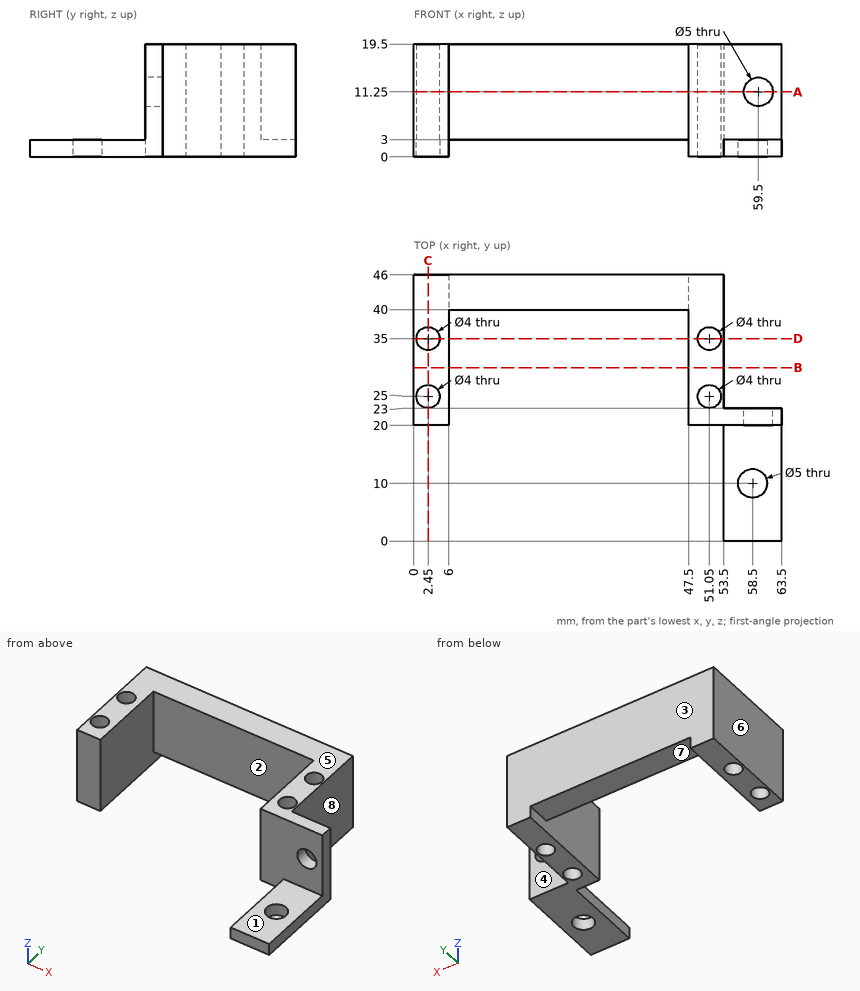
Could you check a few things on this drawing? It's one solid part, dimensions in mm from its lowest x, y, z. A direction names the side the tool comes from. Round coordinates to 2 decimals unless told otherwise and drop trailing zeros. Order: outer loops, then holes, each group sorted by start corner. A loop starts at its lowest first (then second) coordinate and runs counter-clockwise, first axis right, second up. Notation, with made-up numbers: M 5,-24 L 49,-24 A35 cw 49,8 Z; hole C 57.5,18.25 d8. An arc over 180 degrees is marked long. Use a Markdown table: item, result.
1) Imagine slicing it at B-B (y = 30). List the corners of the cut face in (x, z) for me, then the cut area to 3 significant figures.
Geometry says:
| item | result |
|---|---|
| outline | M 0,0 L 6,0 L 6,19.5 L 0,19.5 Z; M 47.5,0 L 53.5,0 L 53.5,19.5 L 47.5,19.5 Z |
| area | 234 mm² |
2) On a 3-axis mill with a long thin cutter (end or side, diameter ignored), from which of +Z, -Z, +X, -X, +Y, -Y can I reach the whole of each face in a straight line? I mean the marked faces 1, 2, 3 and 4. Say none if no direction works.
Geometry says:
| item | result |
|---|---|
| face 1 | +Z, +X, -X, -Y |
| face 2 | +Z, -Z, -Y |
| face 3 | +Z, -Z, +X, -X, +Y |
| face 4 | +Z, -Z, +X, +Y |
3) I'm going to push flat-ended pins straight in: P1, Ø6, axis at x = 17.5, z = 4.5, coming from the -Y side; P2, Ø6.5, axis at x = 30, y = 44, coming from the -Z side; P3, Ø1.8, axis at x = 2.5, z = 9.5, coming from the -Y side. Where does each tip first touch, or does it pass through?
Geometry says:
| item | result |
|---|---|
| P1 | stops at y = 40 |
| P2 | stops at z = 3 |
| P3 | stops at y = 20 |
4) If I drill on line 1 along Y through (x, z) = (2.45, 4.5); line 2 along X through (y, z) = (21.25, 11.25); line 3 along Y through (x, z) = (49, 11), over which ranges is the centre line in solid material (lowest first)?
Geometry says:
| item | result |
|---|---|
| line 1 | y = 20 to 23, 27 to 33, 37 to 46 |
| line 2 | x = 0 to 6, 47.5 to 57, 62 to 63.5 |
| line 3 | y = 20 to 46 |
5) Imagine slicing it at C-C (x = 2.45). List the corners of the cut face in (y, z) for me, then the cut area to 3 significant figures.
Geometry says:
| item | result |
|---|---|
| outline | M 20,0 L 23,0 L 23,19.5 L 20,19.5 Z; M 27,0 L 33,0 L 33,19.5 L 27,19.5 Z; M 37,0 L 46,0 L 46,19.5 L 37,19.5 Z |
| area | 351 mm² |
6) Imagine slicing it at D-D (y = 35). List the corners of the cut face in (x, z) for me, then the cut area to 3 significant figures.
Geometry says:
| item | result |
|---|---|
| outline | M 0,0 L 0.45,0 L 0.45,19.5 L 0,19.5 Z; M 4.45,0 L 6,0 L 6,19.5 L 4.45,19.5 Z; M 47.5,0 L 49.05,0 L 49.05,19.5 L 47.5,19.5 Z; M 53.05,0 L 53.5,0 L 53.5,19.5 L 53.05,19.5 Z |
| area | 78.0 mm² |
7) If we mould it in two halves opening along X, with no side actions, what happens to the marked faces 5, 6, 7 and 8? For each: +X half, -X half, draft (parallel to the pull), parting line (faces both ways), or undercut.
Geometry says:
| item | result |
|---|---|
| face 5 | draft |
| face 6 | -X half |
| face 7 | undercut |
| face 8 | +X half |
8) Imagine slicing it at A-A (z = 11.25). List the corners of the cut face in (x, y) for me.
Geometry says:
| item | result |
|---|---|
| outline | M 0,20 L 6,20 L 6,40 L 47.5,40 L 47.5,20 L 57,20 L 57,23 L 53.5,23 L 53.5,46 L 0,46 Z; M 62,20 L 63.5,20 L 63.5,23 L 62,23 Z; hole C 2.45,25 d4; hole C 2.45,35 d4; hole C 51.05,25 d4; hole C 51.05,35 d4 |
